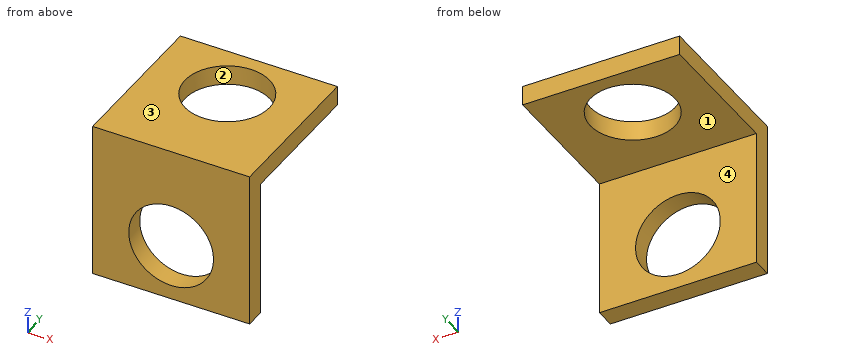
from build123d import *

# Parameters (mm, degrees)
BOSS_EXTRUDE1_DEPTH = 12.7
SKETCH2_R           = 3.429
CUT_EXTRUDE1_DEPTH  = 13.7
SKETCH3_R           = 3.429
CUT_EXTRUDE2_DEPTH  = 13.7


with BuildPart() as part:
    # Sketch1 → Boss-Extrude1 (new body)
    with BuildSketch(Plane(origin=(0, 0, 0), x_dir=(0, 0, -1), z_dir=(1, 0, 0))):
        Polygon((0, 0), (0, 12.7), (1.5875, 12.7), (1.5875, 1.5875), (12.7, 1.5875), (12.7, 0), align=None)
    extrude(amount=BOSS_EXTRUDE1_DEPTH)

    # Sketch2 → Cut-Extrude1 (cut, through all)
    with BuildSketch(Plane.XY):
        with Locations((6.35, 8.128)):
            Circle(SKETCH2_R)
    extrude(amount=-CUT_EXTRUDE1_DEPTH, mode=Mode.SUBTRACT)

    # Sketch3 → Cut-Extrude2 (cut, through all)
    with BuildSketch(Plane.XZ):
        with Locations((6.35, -8.128)):
            Circle(SKETCH3_R)
    extrude(amount=-CUT_EXTRUDE2_DEPTH, mode=Mode.SUBTRACT)


solid = part.part
Work out the finished part from the listing and answer in its coordinate system (mm). Face numbers are marked on the shaded views. A direction names the side the tool comes from. Round coordinates to 2 decimals unless told otherwise and drop trailing zeros. Loops run counter-clockwise (first coordinate to the right, second up) from the corner with the lowest first, then second, coordinate; pieces in that order, holes last. Notation, with made-up numbers: (35.5, 59) - (66.5, 59) arc R29 cw to (66.5, 92) - close; hole circle Ø6 at (82.5, 42.5). An arc over 180 degrees is marked (long way). One line per item, written item: value.
Q1. Find section A-A on x = 6.35. Give the vertices of the cut face in (y, z).
Check values:
outline: (0, -12.7) - (1.59, -12.7) - (1.59, -11.56) - (0, -11.56) - close; (0, -4.7) - (1.59, -4.7) - (1.59, -1.59) - (4.7, -1.59) - (4.7, 0) - (0, 0) - close; (11.56, -1.59) - (12.7, -1.59) - (12.7, 0) - (11.56, 0) - close
Q2. For the marked faces 3 and 4, determine the directions among +Z, -Z, +X, -X, +Y, -Y from which every point of the face is accessible in a straight line to the end or side of a thin tool.
Check values:
face 3: +Z, +X, -X, +Y, -Y
face 4: -Z, +X, -X, +Y
Q3. Find section B-B on z = -7.75. Give the vertices of the cut face in (x, y), and give its area (3 significant figures).
Check values:
outline: (0, 0) - (2.94, 0) - (2.94, 1.59) - (0, 1.59) - close; (9.76, 0) - (12.7, 0) - (12.7, 1.59) - (9.76, 1.59) - close
area: 9.34 mm2
Q4. Find section C-C on y = 9.75. Give the vertices of the cut face in (x, z), and give its area (3 significant figures).
Check values:
outline: (0, -1.59) - (3.33, -1.59) - (3.33, 0) - (0, 0) - close; (9.37, -1.59) - (12.7, -1.59) - (12.7, 0) - (9.37, 0) - close
area: 10.6 mm2
Q5. Find section D-D on x = 3.5. Give the vertices of the cut face in (y, z), and give its area (3 significant figures).
Check values:
outline: (0, -12.7) - (1.59, -12.7) - (1.59, -10.03) - (0, -10.03) - close; (0, -6.22) - (1.59, -6.22) - (1.59, -1.59) - (6.22, -1.59) - (6.22, 0) - (0, 0) - close; (10.03, -1.59) - (12.7, -1.59) - (12.7, 0) - (10.03, 0) - close
area: 25.7 mm2
Q6. Each of these flat-tipped pins is pushed along its axis until it touches: pin 1 Ø4 at (x, z) = (7.5, -8.5) entering from -Y; pin 2 Ø4 at (y, z) = (4.5, -2) entering from +X; pin 3 Ø3.5 at (x, y) = (8.5, 10) entering from -Z. Where does it stop, or does it pass through?
Check values:
pin 1: through
pin 2: x = 12.7
pin 3: z = -1.59
Q7. The mould has two halves that part along X. Classify the marked faces 1 and 2: +X half, -X half, draft (parallel to the pull), parting line (faces both ways), or undercut.
Check values:
face 1: draft
face 2: undercut
Q8. Straight lines are drawn through the part: probe 1 along Y at (x, z) = (6.35, -0.5); probe 2 along Z at (x, y) = (6.35, 0.85); probe 3 along Y at (x, z) = (8, -4). For each, find the intervals that lie inside material, in ascending order.
Check values:
probe 1: 0 to 4.7, 11.56 to 12.7
probe 2: -12.7 to -11.56, -4.7 to 0
probe 3: 0 to 1.59
